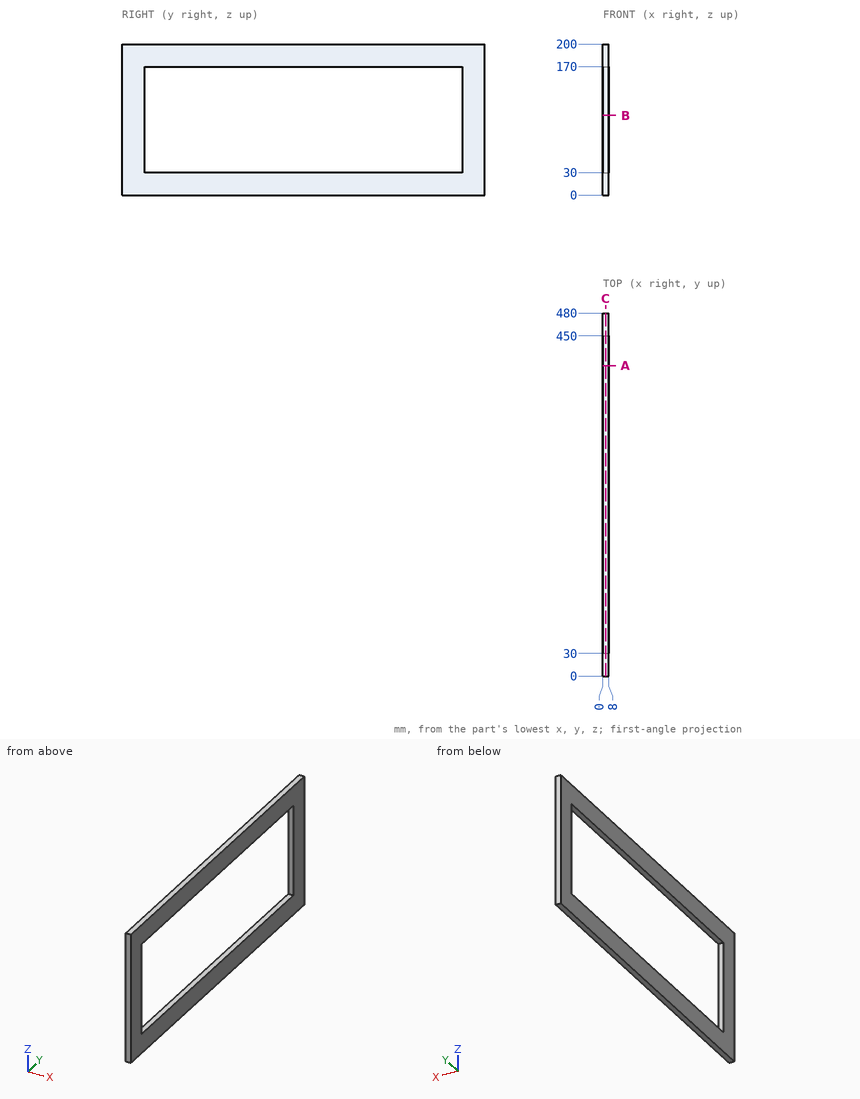
Input: dimensioned drawing with shaded views. Units: mm. Origin: part minimum x, y, z. Round coordinates to 2 decimals unless told otherwise and drop trailing zeros. Order: outer loops, then holes, each group sorted by start corner. A loop starts at its lowest first (then second) coordinate and runs counter-clockwise, first axis right, second up. Notation, with made-up numbers: (78.5, 30.25) - (89.5, 30.25) arc R31 ccw to (89.5, 59.25) - close; hole circle Ø7 at (42, 15.5). An arc over 180 degrees is marked (long way). Answer as a JSON object with one key per item and string values. Group by question number.
(1) Cut plane B-B (z = 105.5). Return loops of the section in (x, y), then the cut area to 3 significant figures.
(2) Material intervals for probe 1 along Y at (x, z) = (7, 32); probe 2 along Z at (x, y) = (3, 150.5), sorted ascending. Write a range as from..to.
(3) Cut plane A-A (y = 410.5). Return loops of the section in (x, z).
(4) Cut plane C-C (x = 3.75). Return loops of the section in (y, z), then the cut area to 3 significant figures.
Here are the results:
{
 "1": {"outline": "(0, 0) - (8, 0) - (8, 30) - (0, 30) - close; (0, 450) - (8, 450) - (8, 480) - (0, 480) - close", "area": "480 mm^2"},
 "2": {"probe 1": "y = 0..30, 450..480", "probe 2": "z = 0..30, 170..200"},
 "3": {"outline": "(0, 0) - (8, 0) - (8, 30) - (0, 30) - close; (0, 170) - (8, 170) - (8, 200) - (0, 200) - close"},
 "4": {"outline": "(0, 0) - (480, 0) - (480, 200) - (0, 200) - close; hole (30, 30) - (450, 30) - (450, 170) - (30, 170) - close", "area": "37,200 mm^2"}
}
